```python
from build123d import *

# Parameters (mm, degrees)
SKETCH_R     = 2
PAD_DEPTH    = 4
CHAMFER_SIZE = 1.5
SKETCH001_R  = 3.5
PAD001_DEPTH = 6
SKETCH002_R  = 3.5
PAD002_DEPTH = 2
FILLET_R     = 1.25


with BuildPart() as part:
    # Sketch → Pad (new body)
    with BuildSketch(Plane.XY):
        with BuildLine():
            Line((-10.5, 0), (-10.5, -20))
            Line((-10.5, -20), (-20.5, -20))
            Line((-20.5, -20), (-20.5, 0))
            ThreePointArc((20.5, 0), (0, 20.5), (-20.5, 0))
            Line((20.5, 0), (20.5, -20))
            Line((20.5, -20), (10.5, -20))
            Line((10.5, -20), (10.5, 0))
            ThreePointArc((10.5, 0), (0, 10.5), (-10.5, 0))
        make_face()
        with Locations((-15.5, 0)):
            Circle(SKETCH_R, mode=Mode.SUBTRACT)
        with Locations((15.5, 0)):
            Circle(SKETCH_R, mode=Mode.SUBTRACT)
    extrude(amount=PAD_DEPTH)

    # Chamfer
    chamfer_edges = [part.edges().sort_by_distance(p)[0] for p in [
        (13.5, 0, 4),
        (-17.5, 0, 4),
    ]]
    chamfer(chamfer_edges, length=CHAMFER_SIZE)

    # Sketch001 (on Face4 of Chamfer) → Pad001 (join)
    with BuildSketch(Plane.XY.offset(4)):
        with BuildLine():
            Line((-10.5, -20), (-20.5, -20))
            Line((-20.5, -20), (-20.5, 0))
            ThreePointArc((20.5, 0), (0, 20.5), (-20.5, 0))
            Line((20.5, -20), (20.5, 0))
            Line((10.5, -20), (20.5, -20))
            Line((10.5, 0), (10.5, -20))
            ThreePointArc((10.5, 0), (0, 10.5), (-10.5, 0))
            Line((-10.5, -20), (-10.5, 0))
        make_face()
        with Locations((-15.5, 0)):
            Circle(SKETCH001_R, mode=Mode.SUBTRACT)
        with Locations((15.5, 0)):
            Circle(SKETCH001_R, mode=Mode.SUBTRACT)
    extrude(amount=PAD001_DEPTH)

    # Sketch002 (on Face14 of Pad001) → Pad002 (join)
    with BuildSketch(Plane.XY.offset(10)):
        with BuildLine():
            Line((-20.5, -20), (20.5, -20))
            Line((20.5, -20), (20.5, 0))
            ThreePointArc((20.5, 0), (0, 20.5), (-20.5, 0))
            Line((-20.5, 0), (-20.5, -20))
        make_face()
        with Locations((-15.5, 0)):
            Circle(SKETCH002_R, mode=Mode.SUBTRACT)
        with Locations((15.5, 0)):
            Circle(SKETCH002_R, mode=Mode.SUBTRACT)
    extrude(amount=PAD002_DEPTH)

    # Fillet
    fillet_edges = [part.edges().sort_by_distance(p)[0] for p in [
        (-20.5, -20, 2),
        (-20.5, -20, 7),
        (-20.5, -20, 11),
        (-20.5, -10, 12),
        (0, 20.5, 12),
        (0, -20, 12),
        (20.5, -10, 12),
        (20.5, -20, 11),
        (20.5, -20, 7),
        (20.5, -20, 2),
    ]]
    fillet(fillet_edges, radius=FILLET_R)


solid = part.part
```
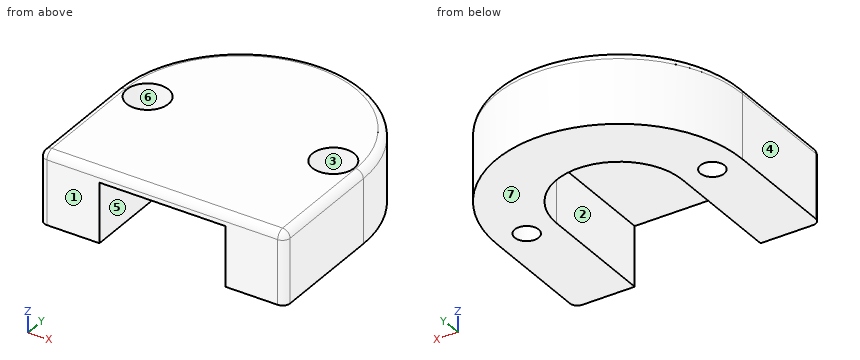
Build history of the part. All positions in model axes, mm. Face numbers are marked on the shaded views. A direction names the side the tool comes from. Coordinates: 2 decimals unless noted, no trailing zeros. Write each loop counter-clockwise with the first axis right and the second up, starting at its lowest first coordinate (ties: lowest second). Pieces come first, ordered by that corner, then holes.
1. Band-saw the part on B-B, the plane y = -16. Give the cut face in (x, z), and give its area (3 significant figures).
Answer block:
outline: (-20.5, 0) - (-10.5, 0) - (-10.5, 10) - (10.5, 10) - (10.5, 0) - (20.5, 0) - (20.5, 10.75) arc R1.25 ccw to (19.25, 12) - (-19.25, 12) arc R1.25 ccw to (-20.5, 10.75) - close
area: 281 mm2
2. Drop flat-ended pins along their axis: pin 1 (4 mm diameter, centred on x = -10.5, z = 2, fed in from +Y); pin 2 (4 mm diameter, centred on x = -16, z = 7, fed in from +Y) (3 decimals); pin 3 (5 mm diameter, centred on y = 4, z = 3.5, fed in from -X). Give the stop position or say it passes through.
Answer block:
pin 1: stops at y = 18.65
pin 2: stops at y = 14.975
pin 3: stops at x = -20.45
3. Band-saw the part on C-C, the plane z = 1. Give the cut face in (x, y).
Answer block:
outline: (-20.5, -18.75) arc R1.25 ccw to (-19.25, -20) - (-10.5, -20) - (-10.5, 0) arc R10.5 cw to (10.5, 0) - (10.5, -20) - (19.25, -20) arc R1.25 ccw to (20.5, -18.75) - (20.5, 0) arc R20.5 ccw to (-20.5, 0) - close; hole circle Ø4 at (-15.5, 0); hole circle Ø4 at (15.5, 0)
4. Band-saw the part on A-A, the plane z = 4.5. Give the cut face in (x, y), and give its area (3 significant figures).
Answer block:
outline: (-20.5, -18.75) arc R1.25 ccw to (-19.25, -20) - (-10.5, -20) - (-10.5, 0) arc R10.5 cw to (10.5, 0) - (10.5, -20) - (19.25, -20) arc R1.25 ccw to (20.5, -18.75) - (20.5, 0) arc R20.5 ccw to (-20.5, 0) - close; hole circle Ø7 at (-15.5, 0); hole circle Ø7 at (15.5, 0)
area: 809 mm2
5. Drill centre lines: probe 1 along X at (y, z) = (-17, 4); probe 2 along Z at (x, y) = (2, 10); probe 3 along X at (y, z) = (8, 7.25). Where is each one in solid material? Low to high.
Answer block:
probe 1: x = -20.5 to -10.5, 10.5 to 20.5
probe 2: z = 10 to 12
probe 3: x = -18.87 to -6.8, 6.8 to 18.87
6. 3-axis set-ups, long thin cutter, end or side, ignore diameter. For the marked faces 1, 2 and 3: which of +Z, -Z, +X, -X, +Y, -Y reach the whole face in a straight line?
Answer block:
face 1: +Z, -Z, +X, -X, -Y
face 2: -Z, -Y
face 3: +Z
7. Pull direction X, two halves, no side cores. Call the marked faces 4, 5, 6 and 7: released by +X, released by -X, zero draft, split by the parting line, or undercut.
Answer block:
face 4: released by -X
face 5: undercut
face 6: undercut
face 7: zero draft
8. Band-saw the part on D-D, the plane y = 0.5. Give the number of separate pieces and of enclosed holes in the cut face, and give its area (3 significant figures).
Answer block:
separate pieces: 3
enclosed holes: 0
area: 135 mm2
